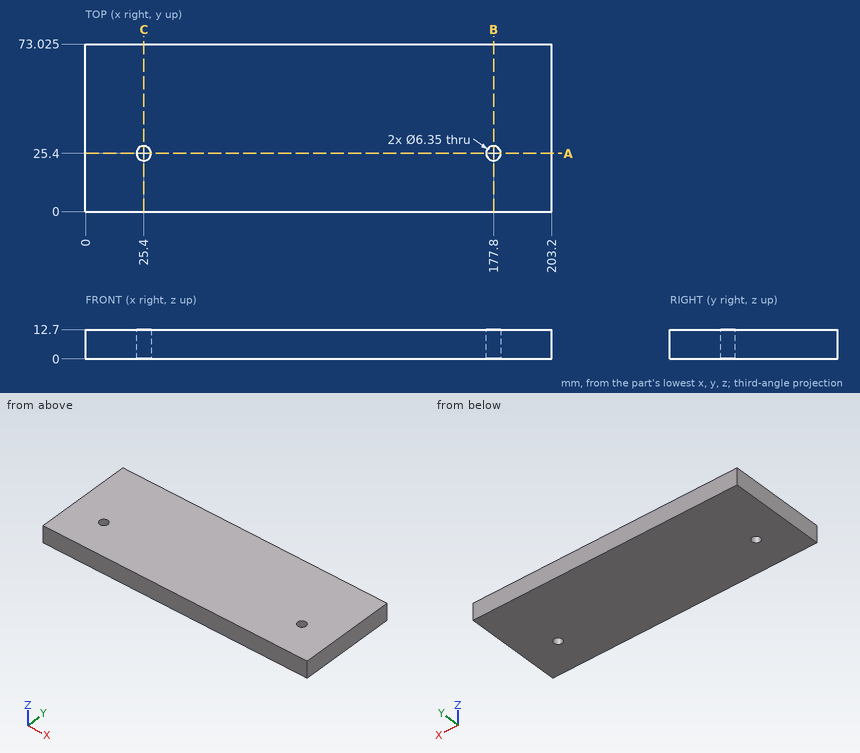
Verification items for this drawing (mm, ordinates from the low corner). Round coordinates to 2 decimals unless told otherwise and drop trailing zeros. Write each loop counter-clockwise with the first axis right and the second up, starting at its lowest first coordinate (ties: lowest second). Pieces come first, ordered by that corner, then holes. Notation, with made-up numbers: M 70,46.25 L 90,46.25 A21 ccw 90,50.25 Z; hole C -30,45.25 d2. An arc over 180 degrees is marked long. Write item = value, one per line. Start each with the question number.
1. Section check A-A, the plane y = 25.4. Record the cut outline in (x, z) (3 decimals).
2. Section check B-B, the plane x = 177.8. Record the cut outline in (y, z) (3 decimals).
3. Scan lines: line 1 (Y direction, x = 177.8, z = 3.75) (3 decimals); line 2 (Y direction, x = 25, z = 11) (3 decimals). Record each from-to range of solid material in increasing order. Write a range as [from, to].
Results found:
q1.outline = M 0,0 L 22.225,0 L 22.225,12.7 L 0,12.7 Z; M 28.575,0 L 174.625,0 L 174.625,12.7 L 28.575,12.7 Z; M 180.975,0 L 203.2,0 L 203.2,12.7 L 180.975,12.7 Z
q2.outline = M 0,0 L 22.225,0 L 22.225,12.7 L 0,12.7 Z; M 28.575,0 L 73.025,0 L 73.025,12.7 L 28.575,12.7 Z
q3.line_1 = [0, 22.225], [28.575, 73.025]
q3.line_2 = [0, 22.25], [28.55, 73.025]
